CAD build for the part. Positions are in the model's coordinates, mm. Face numbers are marked on the shaded views. A direction names the side the tool comes from. Give positions to 0.01 mm unless a question says otherwise; leave off trailing zeros. Write each loop counter-clockwise with the first axis right and the second up, starting at its lowest first coordinate (ties: lowest second). Pieces come first, ordered by that corner, then holes. Notation, with made-up numbers: (-25.75, 75) -> (5.25, 75) arc R11 ccw to (5.25, 79) -> close; hole circle Ø1 at (49, 70). An arc over 180 degrees is marked (long way). Answer as a JSON object with one key per item and string values.
```python
from build123d import *

# Parameters (mm, degrees)
F1_DEPTH = 63.5
F2_DEPTH = 25.4
F3_DEPTH = 7.9375
F5_R     = 6.35


with BuildPart() as f1:
    # F0 (on Front) → F1 (new body, symmetric)
    with BuildSketch(Plane.XZ):
        Polygon((-41.275, -9.525), (41.275, -9.525), (41.275, 9.525), (22.225, 9.525), (-41.275, 9.525), align=None)
    extrude(amount=F1_DEPTH, both=True)

    # F0 (on Front) → F2 (join, symmetric)
    with BuildSketch(Plane.XZ):
        with BuildLine():
            Line((22.225, 9.525), (41.275, 9.525))
            Line((41.275, 9.525), (41.275, 27.0002))
            ThreePointArc((41.275, 27.0002), (45.92468, 38.22552), (57.15, 42.8752))
            Line((57.15, 42.8752), (60.325, 42.8752))
            Line((60.325, 42.8752), (60.325, 61.9252))
            Line((60.325, 61.9252), (57.15, 61.9252))
            ThreePointArc((57.15, 61.9252), (32.454296, 51.695904), (22.225, 27.0002))
            Line((22.225, 27.0002), (22.225, 9.525))
        make_face()
        Polygon((85.725, 61.9252), (60.325, 61.9252), (60.325, 42.8752), (85.702203, 42.8752), align=None)
    extrude(amount=F2_DEPTH, both=True)

    # F0 (on Front) → F3 (join, symmetric)
    with BuildSketch(Plane.XZ):
        with BuildLine():
            add(Edge.make_bspline(
                [(-41.275, 9.525), (-25.517739, 36.63322), (3.348505, 62.103435), (57.15, 61.9252)],
                knots=[0, 0, 0, 0, 111.504536, 111.504536, 111.504536, 111.504536], degree=3))
            Line((-41.275, 9.525), (22.225, 9.525))
            Line((22.225, 9.525), (22.225, 27.0002))
            ThreePointArc((22.225, 27.0002), (32.454296, 51.695904), (57.15, 61.9252))
        make_face()
    extrude(amount=F3_DEPTH, both=True)

    # F0 (on Front) → F4 (revolve)
    with BuildSketch(Plane.XZ):
        Polygon((85.725, 66.675), (85.725, 61.9252), (85.725, 38.1), (111.125, 38.1), (111.125, 66.675), align=None)
    revolve(axis=Axis((85.725, 0, 52.3875), (0, 0, -1)))

    # F5
    f5_edges = [f1.edges().sort_by_distance(p)[0] for p in [
        (41.275, -63.5, 0),
        (41.275, 63.5, 0),
        (-41.275, -63.5, 0),
        (-41.275, 63.5, 0),
    ]]
    fillet(f5_edges, radius=F5_R)


solid = f1.part
```
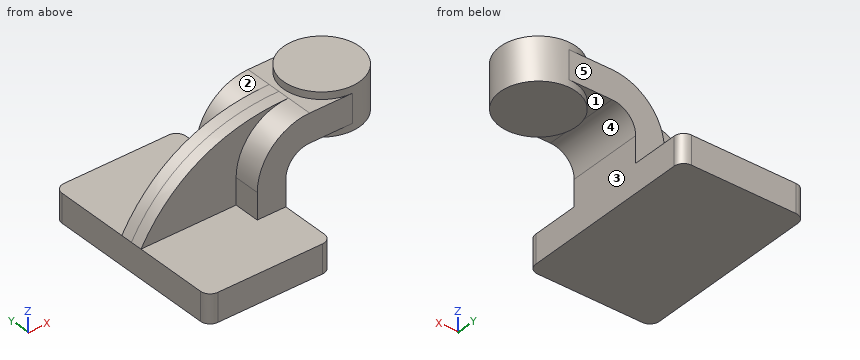
1) Pin check, flat tips, straight feed: pin 1 (1.5 mm diameter, centred on x = 24, z = 21.5, fed in from +Y); pin 2 (10 mm diameter, centred on x = 22, z = 37.5, fed in from -Y); pin 3 (2 mm diameter, centred on x = 18.5, z = 56, fed in from +Y); pin 4 (12 mm diameter, centred on x = 61, y = -35, fed in from -Z). Stop position of each tip, or through.
Model answer:
{"pin 1": "stops at y = 25.4", "pin 2": "stops at y = -25.4", "pin 3": "stops at y = 7.94", "pin 4": "passes through"}
2) Slice it at B-B (y = 40). List the corners of the cut face in (x, z) (3 decimals).
Model answer:
{"outline": "(-41.275, -9.525) -> (41.275, -9.525) -> (41.275, 9.525) -> (-41.275, 9.525) -> close"}
3) 3-axis set-ups, long thin cutter, end or side, ignore diameter. For the marked faces 1, 2, 3, 4 and 5: which of +Z, -Z, +X, -X, +Y, -Y reach the whole face in a straight line?
Model answer:
{"face 1": "-Z", "face 2": "+Z, -X, +Y", "face 3": "-Z, +X, +Y, -Y", "face 4": "-Z, +Y, -Y", "face 5": "+Z, +X, -X, +Y"}
4) Slice it at A-A (y = 16). List the corners of the cut face in (x, z) (3 decimals), then the cut area to 3 significant figures.
Model answer:
{"outline": "(-41.275, -9.525) -> (41.275, -9.525) -> (41.275, 27) arc R15.875 cw to (57.15, 42.875) -> (65.998, 42.875) -> (65.998, 38.1) -> (105.452, 38.1) -> (105.452, 66.675) -> (65.998, 66.675) -> (65.998, 61.925) -> (57.15, 61.925) arc R34.925 ccw to (22.225, 27) -> (22.225, 9.525) -> (-41.275, 9.525) -> close", "area": "3,960 mm2"}
5) Wall check: probe 1 along Z at (x, y) = (19, -19) (3 decimals); probe 2 along Z at (x, y) = (83, 3) (3 decimals); probe 3 along Y at (x, z) = (20, 26). Give the ranges that are in metal, low to high.
Model answer:
{"probe 1": "z = -9.525 to 9.525", "probe 2": "z = 38.1 to 66.675", "probe 3": "y = -7.94 to 7.94"}
